from build123d import *

# Parameters (mm, degrees)
SKETCH1_R                                       = 1
SKETCH1_R_2                                     = 2.7
BOSS_EXTRUDE1_DEPTH                             = 6
FILLET1_R                                       = 7.5
SKETCH2_R                                       = 1.6
CUT_EXTRUDE1_DEPTH                              = 66.108380797
SKETCH3_OUTSIDE_W                               = 133.41
SKETCH3_OUTSIDE_H                               = 103.41
SKETCH3_OUTSIDE_R                               = 30.525
CUT_EXTRUDE3_DEPTH                              = 1.25
CSK_FOR_M3_FLAT_HEAD_MACHINE_SCREW1_D           = 3.4
CSK_FOR_M3_FLAT_HEAD_MACHINE_SCREW1_CSINK_D     = 6.3
CSK_FOR_M3_FLAT_HEAD_MACHINE_SCREW1_CSINK_ANGLE = 90


with BuildPart() as part:
    # Sketch1 → Boss-Extrude1 (new body)
    with BuildSketch(Plane(origin=(0, 0, 0), x_dir=(1, 0, 0), z_dir=(0, 1, 0))):
        with BuildLine():
            Line((31.883633055, 20.164562188), (44.561021943, 28.182280752))
            ThreePointArc((44.561021943, 28.182280752), (52.725, 0), (44.561021943, -28.182280752))
            Line((44.561021943, -28.182280752), (31.883633055, -20.164562188))
            ThreePointArc((31.883633055, -20.164562188), (0, -37.725), (-31.883633055, -20.164562188))
            Line((-31.883633055, -20.164562188), (-44.561021943, -28.182280752))
            ThreePointArc((-44.561021943, -28.182280752), (-52.725, 0), (-44.561021943, 28.182280752))
            Line((-44.561021943, 28.182280752), (-31.883633055, 20.164562188))
            ThreePointArc((-31.883633055, 20.164562188), (0, 37.725), (31.883633055, 20.164562188))
        make_face()
        with Locations(Location((-13.0112367, 31.411904105, 0), (0, 0, 270))):
            Circle(SKETCH1_R, mode=Mode.SUBTRACT)
        with Locations(Location((13.0112367, 31.411904105, 0), (0, 0, 270))):
            Circle(SKETCH1_R, mode=Mode.SUBTRACT)
        with Locations(Location((31.411904105, 13.0112367, 0), (0, 0, 270))):
            Circle(SKETCH1_R, mode=Mode.SUBTRACT)
        with Locations(Location((31.411904105, -13.0112367, 0), (0, 0, 270))):
            Circle(SKETCH1_R, mode=Mode.SUBTRACT)
        with Locations(Location((13.0112367, -31.411904105, 0), (0, 0, 270))):
            Circle(SKETCH1_R, mode=Mode.SUBTRACT)
        with Locations(Location((-13.0112367, -31.411904105, 0), (0, 0, 270))):
            Circle(SKETCH1_R, mode=Mode.SUBTRACT)
        with Locations(Location((-31.411904105, -13.0112367, 0), (0, 0, 270))):
            Circle(SKETCH1_R, mode=Mode.SUBTRACT)
        with Locations(Location((-31.411904105, 13.0112367, 0), (0, 0, 270))):
            Circle(SKETCH1_R, mode=Mode.SUBTRACT)
        with Locations(Location((41.701925915, 17.5, 0), (0, 0, 270))):
            Circle(SKETCH1_R_2, mode=Mode.SUBTRACT)
        with Locations(Location((41.701925915, -17.5, 0), (0, 0, 270))):
            Circle(SKETCH1_R_2, mode=Mode.SUBTRACT)
        with Locations(Location((-41.701925915, 17.5, 0), (0, 0, 90))):
            Circle(SKETCH1_R_2, mode=Mode.SUBTRACT)
        with Locations(Location((-41.701925915, -17.5, 0), (0, 0, 90))):
            Circle(SKETCH1_R_2, mode=Mode.SUBTRACT)
    extrude(amount=BOSS_EXTRUDE1_DEPTH)

    # Fillet1
    fillet1_edges = [part.edges().sort_by_distance(p)[0] for p in [
        (44.561021943, 3, 28.182280752),
        (31.883633055, 3, 20.164562188),
        (-44.561021943, 3, 28.182280752),
        (-31.883633055, 3, 20.164562188),
        (44.561021943, 3, -28.182280752),
        (31.883633055, 3, -20.164562188),
        (-44.561021943, 3, -28.182280752),
        (-31.883633055, 3, -20.164562188),
    ]]
    fillet(fillet1_edges, radius=FILLET1_R - 0.0001)  # a hair under: the kernel refuses the full size

    # Sketch2 → Cut-Extrude1 (cut, through all)
    with BuildSketch(Plane(origin=(0, 6, 0), x_dir=(1, 0, 0), z_dir=(0, 1, 0))):
        with Locations(Location((0, 34, 0), (0, 0, 270))):
            Circle(SKETCH2_R)
    extrude(amount=-CUT_EXTRUDE1_DEPTH, mode=Mode.SUBTRACT)

    # Sketch3 outside → Cut-Extrude3 (cut)
    with BuildSketch(Plane(origin=(0, 6, 0), x_dir=(1, 0, 0), z_dir=(0, 1, 0))):
        Rectangle(SKETCH3_OUTSIDE_W, SKETCH3_OUTSIDE_H)
        with Locations(Location((0, 0, 0), (0, 0, 270))):
            Circle(SKETCH3_OUTSIDE_R, mode=Mode.SUBTRACT)
    extrude(amount=-CUT_EXTRUDE3_DEPTH, mode=Mode.SUBTRACT)

    # CSK for M3 Flat Head Machine Screw1 (through all)
    with Locations(Plane(origin=(0, 0, 0), x_dir=(-1, 0, 0), z_dir=(0, -1, 0))):
        with Locations((13.0112367, -31.411904105), (-13.0112367, -31.411904105), (-31.411904105, -13.0112367), (-31.411904105, 13.0112367), (-13.0112367, 31.411904105), (13.0112367, 31.411904105), (31.411904105, 13.0112367), (31.411904105, -13.0112367)):
            CounterSinkHole(CSK_FOR_M3_FLAT_HEAD_MACHINE_SCREW1_D / 2, CSK_FOR_M3_FLAT_HEAD_MACHINE_SCREW1_CSINK_D / 2, counter_sink_angle=CSK_FOR_M3_FLAT_HEAD_MACHINE_SCREW1_CSINK_ANGLE)


solid = part.part
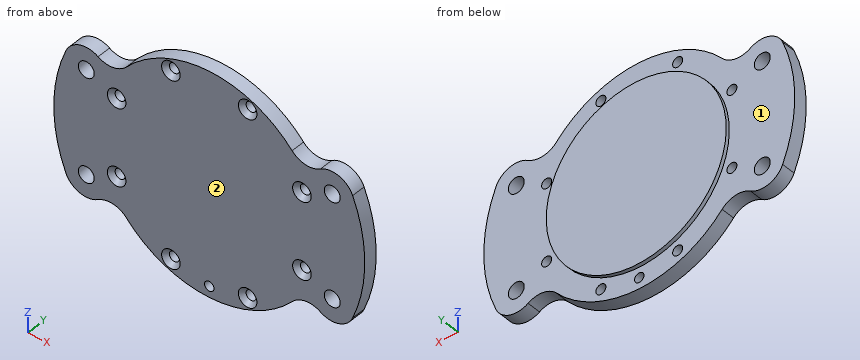
Read the model definition and answer for the solid it produces. Units are mm, in the model's axes. Face numbers are marked on the shaded views. A direction names the side the tool comes from. Round coordinates to 2 decimals unless told otherwise and drop trailing zeros. Write each loop counter-clockwise with the first axis right and the second up, starting at its lowest first coordinate (ties: lowest second). Pieces come first, ordered by that corner, then holes. Notation, with made-up numbers: (-13, 33.5) - (13, 33.5) arc R22 cw to (13, 47.5) - close; hole circle Ø9 at (-33, 4.5). An arc over 180 degrees is marked (long way). One line per question, with ' | ' between items. Start each with the question number.
1. For the marked faces 1 and 2, determine the directions among +Z, -Z, +X, -X, +Y, -Y from which every point of the face is accessible in a straight line to the end or side of a thin tool.
2. Section B-B (z = -17.5) is taken. Determine the outline of the cut face in (x, y).
3. Find the intervals of material crossed by probe 1 along X at (y, z) = (1.6, -17.5); probe 2 along X at (y, z) = (0.9, -11); probe 3 along Y at (x, z) = (45.5, 16), in increasing order. Write a range as [from, to].
4. Section A-A (y = 3.5) is taken. Give the number of separate pieces and of enclosed holes in the cut face, and give its area (3 significant figures).
5. Section D-D (x = -26.5) is taken. Determine the outline of the cut face in (y, z).
6. Each of these flat-tipped pins is pushed along its axis until it touches: pin 1 (2 mm diameter, centred on x = 6.5, y = 3, fed in from +Z); pin 2 (4 mm diameter, centred on x = -31.41, z = -13.01, fed in from +Y); pin 3 (5.5 mm diameter, centred on x = 13.01, z = 31.41, fed in from -Y). Where does it stop, or does it pass through?
7. Section C-C (z = 2) is taken. Determine the outline of the cut face in (x, y), and give its area (3 significant figures).
Filled in:
1) face 1: +Y | face 2: +Z, -Z, +X, -X, -Y
2) outline: (-49.74, 0) - (-44.4, 0) - (-44.4, 4.75) - (-49.74, 4.75) - close; (-39, 0) - (39, 0) - (39, 4.75) - (25.01, 4.75) - (25.01, 6) - (-25.01, 6) - (-25.01, 4.75) - (-39, 4.75) - close; (44.4, 0) - (49.74, 0) - (49.74, 4.75) - (44.4, 4.75) - close
3) probe 1: [-49.74, -44.4], [-39, 39], [44.4, 49.74] | probe 2: [-51.56, -32.42], [-30.4, 30.4], [32.42, 51.56] | probe 3: [0, 4.75]
4) separate pieces: 1 | enclosed holes: 13 | area: 5,800 mm²
5) outline: (0, -26.85) - (4.75, -26.85) - (4.75, -15.15) - (6, -15.15) - (6, 15.15) - (4.75, 15.15) - (4.75, 26.85) - (0, 26.85) - close
6) pin 1: z = 37.32 | pin 2: y = 4.75 | pin 3: y = 0.4
7) outline: (-52.69, 0) - (52.69, 0) - (52.69, 4.75) - (30.46, 4.75) - (30.46, 6) - (-30.46, 6) - (-30.46, 4.75) - (-52.69, 4.75) - close | area: 577 mm²
